```python
from build123d import *

# Parameters (mm, degrees)
F0_R     = 2.25
F1_DEPTH = 5
F2_SIZE2 = 2.34
F2_SIZE  = 2.137


with BuildPart() as f1:
    # F0 (on Front) → F1 (new body)
    with BuildSketch(Plane.XZ):
        with BuildLine():
            Line((20, 10), (-20, 10))
            ThreePointArc((-20, 10), (-30, 0), (-20, -10))
            Line((-20, -10), (20, -10))
            ThreePointArc((20, -10), (30, 0), (20, 10))
        make_face()
        with Locations((-20, 0)):
            Circle(F0_R, mode=Mode.SUBTRACT)
        with Locations((20, 0)):
            Circle(F0_R, mode=Mode.SUBTRACT)
    extrude(amount=F1_DEPTH)

    # F2
    f2_edges = [f1.edges().sort_by_distance(p)[0] for p in [
        (17.75, -5, 0),
        (-22.25, -5, 0),
    ]]
    chamfer(f2_edges, length=F2_SIZE, length2=F2_SIZE2)


solid = f1.part
```
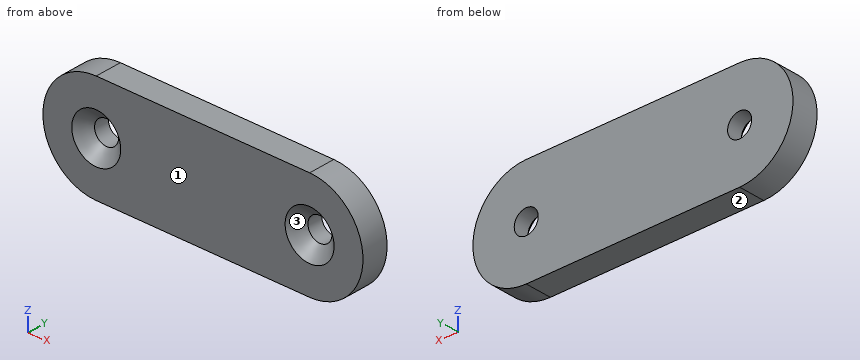
Could you check a few things on this model? Use its own coordinates, in mm. Face numbers are marked on the shaded views. Round coordinates to 2 decimals unless told otherwise and drop trailing zeros. Write each loop counter-clockwise with the first axis right and the second up, starting at its lowest first coordinate (ties: lowest second). Pieces come first, ordered by that corner, then holes. Notation, with made-up numbers: M -29.5,-25.75 L 21.5,-25.75 A33 cw 21.5,2.25 Z; hole C 47,-33.5 d3. An arc over 180 degrees is marked long. Answer in a Markdown table with one row per item. Add a question column.
Q1. Imagine slicing it at D-D (z = -5.5). Please give me the cut outline in (x, y).
Q2. Will this pin go through, and if not, where does the flat tip stop? pin 1 Ø2 at (y, z) = (-4, 1.5) entering from +X.
Q3. Imagine slicing it at A-A (z = 0). Please give me the cut outline in (x, y), then the cut area to 3 significant figures.
Q4. Imagine slicing it at B-B (y = -2.15). Please give me the cut outline in (x, z).
Q5. Imagine slicing it at C-C (z = -8). Please give me the cut outline in (x, y), then the cut area to 3 significant figures.
Q6. If we mould it in two halves opening along Z, with no side actions, what happens to the marked faces 1, 2 and 3? For each: +Z half, -Z half, draft (parallel to the pull), parting line (faces both ways), or undercut.
Q7. If I drill on line 1 (X direction, y = -2.7, z = -2); line 2 (X direction, y = -2.65, z = -0.25); line 3 (Z direction, x = 20, y = -2), over which ranges is the centre line in solid material (lowest first)? Write a range as from..to.
Values:
| question | item | result |
|---|---|---|
| 1 | outline | M -28.35,-5 L 28.35,-5 L 28.35,0 L -28.35,0 Z |
| 2 | pin 1 | x = 29.99 |
| 3 | outline | M -30,-5 L -24.59,-5 L -22.25,-2.86 L -22.25,0 L -30,0 Z; M -17.75,-2.86 L -15.41,-5 L 15.41,-5 L 17.75,-2.86 L 17.75,0 L -17.75,0 Z; M 22.25,-2.86 L 24.59,-5 L 30,-5 L 30,0 L 22.25,0 Z |
| 3 | area | 245 mm^2 |
| 4 | outline | M -20,-10 L 20,-10 A10 ccw 20,10 L -20,10 A10 ccw Z; hole C -20,0 d4.5; hole C 20,0 d4.5 |
| 5 | outline | M -26,-5 L 26,-5 L 26,0 L -26,0 Z |
| 5 | area | 260 mm^2 |
| 6 | face 1 | draft |
| 6 | face 2 | -Z half |
| 6 | face 3 | undercut |
| 7 | line 1 | -29.8..-21.03, -18.97..18.97, 21.03..29.8 |
| 7 | line 2 | -30..-22.24, -17.76..17.76, 22.24..30 |
| 7 | line 3 | -10..-2.25, 2.25..10 |
